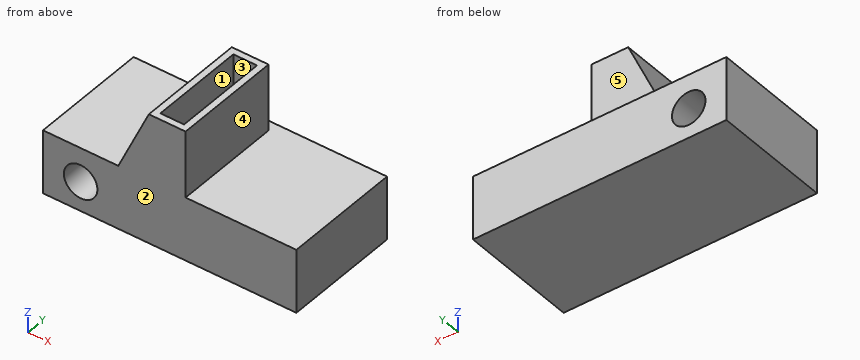
```python
from build123d import *

# Parameters (mm, degrees)
F0_W     = 108.4789782763
F0_H     = 27.2507588379
F1_DEPTH = 50.8
F3_DEPTH = 46.482
F4_R     = 7.1675152866
F5_DEPTH = 50.801
F6_W     = 10.1335914806
F6_H     = 40.894000291
F7_DEPTH = 26.162


with BuildPart() as f1:
    # F0 (on Front) → F1 (new body)
    with BuildSketch(Plane.XZ):
        with Locations((1.3101398945, 20.7000973169)):
            Rectangle(F0_W, F0_H)
    extrude(amount=F1_DEPTH)

    # F2 (on face) → F3 (join)
    with BuildSketch(Plane.XZ.offset(50.8)):
        Polygon((-7.5987614691, 62.886364758), (-20.7000877708, 34.3254767358), (8.1228297204, 34.3254767358), (8.1228297204, 62.886364758), align=None)
    extrude(amount=-F3_DEPTH)

    # F4 (on face) → F5 (cut, through all)
    with BuildSketch(Plane.XZ.offset(50.8)):
        with Locations((-36.8147185072, 19.7747178979)):
            Circle(F4_R)
    extrude(amount=-F5_DEPTH, mode=Mode.SUBTRACT)

    # F6 (on face) → F7 (cut)
    with BuildSketch(Plane.XY.offset(62.886364758)):
        with Locations((0.2620341256, -27.559)):
            Rectangle(F6_W, F6_H)
    extrude(amount=-F7_DEPTH, mode=Mode.SUBTRACT)


solid = f1.part
```
For this review, take the finished solid that the model builds, in its own axes (mm). Face numbers are marked on the shaded views. A direction names the side the tool comes from. Coordinates: 2 decimals unless noted, no trailing zeros. Loops run counter-clockwise (first coordinate to the right, second up) from the corner with the lowest first, then second, coordinate; pieces in that order, holes last.
1. Mouldability with a two-part tool opening along Y and no side actions: class the marked faces 3, 4 and 5 as +Y half, -Y half, draft (parallel to the pull), parting line (faces both ways), or undercut.
2. Insertion check: P1, Ø2, axis at x = -32, y = -17.5, coming from the +Z side; P2, Ø5, axis at y = -34.5, z = 49, coming from the +X side; P3, Ø3, axis at x = -4, z = 47.5, coming from the +Y side. Each pin has a flat end and moves straight along its axis. Give the tip position at first contact, or say it passes through.
3. Add section A-A, the plane z = 15. Give the boundary of the cut face in (x, y).
4. For the marked faces 1 and 2, list the 3-axis set-ups (+Z, -Z, +X, -X, +Y, -Y) from which the entire face can be reached by the end or side of a thin tool; tool diameter is ignored.
5. For line 1 (Z direction, x = 39.5, y = -7); line 2 (Y direction, x = -2, z = 53); line 3 (X direction, y = -19, z = 17), list the stretches that pass through material, from the lowest coordinate up.
6. Add section C-C, the plane x = -40. Give the boundary of the cut face in (y, z), then the cut area to 3 significant figures.
7. Add section D-D, the plane z = 49.5. Give the boundary of the cut face in (x, y), then the cut area to 3 significant figures.
8. Add section B-B, the plane y = -43. Give the boundary of the cut face in (x, z), then the cut area to 3 significant figures.
Result:
1. face 3: undercut
1. face 4: draft
1. face 5: +Y half
2. P1: stops at z = 34.33
2. P2: stops at x = 8.12
2. P3: stops at y = -4.32
3. outline: (-52.93, -50.8) - (-42.16, -50.8) - (-42.16, 0) - (-52.93, 0) - close; (-31.47, -50.8) - (55.55, -50.8) - (55.55, 0) - (-31.47, 0) - close
4. face 1: +Z
4. face 2: +Z, -Z, +X, -X, -Y
5. line 1: z = 7.07 to 34.33
5. line 2: y = -50.8 to -48.01, -7.11 to -4.32
5. line 3: x = -52.93 to -43.42, -30.21 to 55.55
6. outline: (-50.8, 7.07) - (0, 7.07) - (0, 13.35) - (-50.8, 13.35) - close; (-50.8, 26.2) - (0, 26.2) - (0, 34.33) - (-50.8, 34.33) - close
6. area: 732 mm2
7. outline: (-13.74, -50.8) - (8.12, -50.8) - (8.12, -4.32) - (-13.74, -4.32) - close; hole (-4.8, -48.01) - (5.33, -48.01) - (5.33, -7.11) - (-4.8, -7.11) - close
7. area: 602 mm2
8. outline: (-52.93, 7.07) - (55.55, 7.07) - (55.55, 34.33) - (8.12, 34.33) - (8.12, 62.89) - (5.33, 62.89) - (5.33, 36.72) - (-4.8, 36.72) - (-4.8, 62.89) - (-7.6, 62.89) - (-20.7, 34.33) - (-52.93, 34.33) - close; hole circle Ø14.34 at (-36.81, 19.77)
8. area: 3,170 mm2
